Part model, mm, in its own coordinate system. A direction names the side the tool comes from. Round coordinates to 2 decimals unless told otherwise and drop trailing zeros. Write each loop counter-clockwise with the first axis right and the second up, starting at its lowest first coordinate (ties: lowest second). Pieces come first, ordered by that corner, then holes. Notation, with made-up numbers: M 29,32 L 80,32 A25 cw 80,57 Z; hole C -17.75,-20 d7. An arc over 180 degrees is marked long. One line per question, with ' | ' between items. Start each with the question number.
1) Tool access for faces 4 (the face through (-63.86, -11.924, 1.268)), 5 (the face through (-61.36, -7.4, -1.52)), 6 (the face through (-32.733, 21.384, 1.268)): list every direction of +Z, -Z, +X, -X, +Y, -Y with a clear straight run to the whole face (end or side of a thin tool).
2) Drop flat-ended pins along their axis: pin 1 Ø5 at (x, y) = (-45.06, 0.94) entering from +Z; pin 2 Ø3 at (x, y) = (-45.5, 13) entering from -Z; pin 3 Ø1.2 at (x, z) = (-39.5, 1.5) entering from +Y; pin 4 Ø4 at (x, y) = (-36.06, -17.06) entering from +Z. Give the stop position or say it passes through.
3) Saw through at C-C (y = 21). List the corners of the cut face in (x, z).
4) Mould opens along Y. For faces 1 (the face through (-45, 32, 0)), 2 (the face through (-61.36, 21.27, -1.52)), 3 (the face through (-45, -13.064, 1)) say: pulls with the +Y half, pulls with the -Y half, needs draft (parallel to the pull), parting line crosses it, or undercut.
5) Saw through at D-D (x = -48.5). List the corners of the cut face in (y, z), plus the area to 3 significant figures.
6) Saw through at A-A (x = -36). List the corners of the cut face in (y, z), plus the area to 3 significant figures.
7) Saw through at B-B (z = 0.65). List the corners of the cut face in (x, y).
8) Wall check: probe 1 along Y at (x, z) = (-44, -1.25); probe 2 along X at (y, z) = (19.5, -1.15); probe 3 along Y at (x, z) = (-32.5, 0.4). Give the ranges that are in metal, low to high. Write a range as [from, to].
```python
from build123d import *

# Parameters (mm, degrees)
SKETCH_2_W               = 40
SKETCH_2_H               = 40
EXTRUDE_1_DEPTH          = 2.5
SKETCH_5_W               = 40
SKETCH_5_H               = 60
SKETCH_5_R               = 1.5
EXTRUDE_2_DEPTH          = 3
SKETCH_4_R               = 1.5
SKETCH_4_R_2             = 1.10000034
CUT_EXTRUDE_1_DEPTH      = 6.5
FILLET_1_R               = 4
FILLET_5_R               = 2
SKETCH_6_R               = 3
CUT_EXTRUDE_2_DEPTH      = 3
MIRROR_2_COPY_1_SKETCH_R = 3
MIRROR_2_COPY_1_DEPTH    = 3
SKETCH_7_R               = 2
CUT_EXTRUDE_3_DEPTH      = 3


with BuildPart() as part:
    # 草图2 → 凸台-拉伸1 (new body)
    with BuildSketch(Plane.XY):
        with Locations((-45.062828034, 6.935543198)):
            Rectangle(SKETCH_2_W, SKETCH_2_H)
    extrude(amount=EXTRUDE_1_DEPTH)

    # 草图5 → 凸台-拉伸2 (add)
    with BuildSketch(Plane(origin=(0, 0, 0), x_dir=(-1, 0, 0), z_dir=(0, 0, -1))):
        with Locations((45.062828034, 6.935543198)):
            Rectangle(SKETCH_5_W, SKETCH_5_H)
        with Locations((36.062828034, 30.935543198)):
            Circle(SKETCH_5_R, mode=Mode.SUBTRACT)
        with Locations((54.062828034, 30.935543198)):
            Circle(SKETCH_5_R, mode=Mode.SUBTRACT)
        with Locations((54.062828034, -17.064456802)):
            Circle(SKETCH_5_R, mode=Mode.SUBTRACT)
        with Locations((36.062828034, -17.064456802)):
            Circle(SKETCH_5_R, mode=Mode.SUBTRACT)
    extrude(amount=EXTRUDE_2_DEPTH)

    # 草图4 → 切除-拉伸1 (cut, through all)
    with BuildSketch(Plane.XY.offset(2.5)):
        with Locations((-31.627799192, 20.370572041)):
            Circle(SKETCH_4_R)
        with Locations((-58.497856877, 20.370572041)):
            Circle(SKETCH_4_R)
        with Locations((-58.497856877, -6.499485644)):
            Circle(SKETCH_4_R)
        with Locations((-31.627799192, -6.499485644)):
            Circle(SKETCH_4_R)
        with Locations((-45.062828034, 12.935531198)):
            Circle(SKETCH_4_R_2)
        with Locations((-45.062828034, 0.935555198)):
            Circle(SKETCH_4_R_2)
    extrude(amount=-CUT_EXTRUDE_1_DEPTH, mode=Mode.SUBTRACT)

    # 圆角1
    fillet_1_edges = [part.edges().sort_by_distance(p)[0] for p in [
        (-25.062828034, -13.064456802, 1.25),
        (-65.062828034, -13.064456802, 1.25),
        (-65.062828034, 26.935543198, 1.25),
        (-25.062828034, 26.935543198, 1.25),
    ]]
    fillet(fillet_1_edges, radius=FILLET_1_R)

    # 圆角5
    fillet_5_edges = [part.edges().sort_by_distance(p)[0] for p in [
        (-25.062828034, 36.935543198, -1.5),
        (-25.062828034, -23.064456802, -1.5),
        (-65.062828034, -23.064456802, -1.5),
        (-65.062828034, 36.935543198, -1.5),
    ]]
    fillet(fillet_5_edges, radius=FILLET_5_R)

    # 草图6 → 切除-拉伸2 (cut)
    with BuildSketch(Plane(origin=(0, 0, -3), x_dir=(-1, 0, 0), z_dir=(0, 0, -1))):
        with Locations((58.497856877, 20.370572041)):
            Circle(SKETCH_6_R)
    cut_extrude_2 = extrude(amount=-CUT_EXTRUDE_2_DEPTH, mode=Mode.SUBTRACT)

    # 镜向1: 切除-拉伸2 across plane
    add(cut_extrude_2.mirror(Plane.ZX.offset(6.935543198)), mode=Mode.SUBTRACT)

    # 镜向2: 切除-拉伸2 across plane
    add(cut_extrude_2.mirror(Plane.ZY.offset(45.062828034)), mode=Mode.SUBTRACT)

    # 镜向2 copy 1 sketch → 镜向2 copy 1 (cut)
    with BuildSketch(Plane(origin=(-90.125656068, 13.871086397, -3), x_dir=(1, 0, 0), z_dir=(0, 0, -1))):
        with Locations((58.497856877, 20.370572041)):
            Circle(MIRROR_2_COPY_1_SKETCH_R)
    extrude(amount=-MIRROR_2_COPY_1_DEPTH, mode=Mode.SUBTRACT)

    # 草图7 → 切除-拉伸3 (cut)
    with BuildSketch(Plane(origin=(0, 0, -3), x_dir=(-1, 0, 0), z_dir=(0, 0, -1))):
        with Locations((45.062828034, 12.935531198)):
            Circle(SKETCH_7_R)
        with Locations((45.062828034, 0.935555198)):
            Circle(SKETCH_7_R)
    extrude(amount=-CUT_EXTRUDE_3_DEPTH, mode=Mode.SUBTRACT)


solid = part.part
```
Answer key:
1) face 4: +Z, -X, -Y | face 5: -Z | face 6: +Z, -Z
2) pin 1: stops at z = 2.5 | pin 2: stops at z = 0 | pin 3: stops at y = 26.94 | pin 4: stops at z = 0
3) outline: M -65.06,-3 L -61.43,-3 L -61.43,0 L -59.86,0 L -59.86,2.5 L -65.06,2.5 Z; M -57.14,0 L -55.56,0 L -55.56,-3 L -34.56,-3 L -34.56,0 L -32.99,0 L -32.99,2.5 L -57.14,2.5 Z; M -30.27,0 L -28.69,0 L -28.69,-3 L -25.06,-3 L -25.06,2.5 L -30.27,2.5 Z
4) face 1: needs draft | face 2: undercut | face 3: pulls with the -Y half
5) outline: M -23.06,-3 L 36.94,-3 L 36.94,0 L 26.94,0 L 26.94,2.5 L -13.06,2.5 L -13.06,0 L -23.06,0 Z | area: 280 mm2
6) outline: M -23.06,-3 L -18.56,-3 L -18.56,0 L -23.06,0 Z; M -15.57,-3 L 29.44,-3 L 29.44,0 L 26.94,0 L 26.94,2.5 L -13.06,2.5 L -13.06,0 L -15.57,0 Z; M 32.43,-3 L 36.94,-3 L 36.94,0 L 32.43,0 Z | area: 262 mm2
7) outline: M -65.06,-9.06 A4 ccw -61.06,-13.06 L -29.06,-13.06 A4 ccw -25.06,-9.06 L -25.06,22.94 A4 ccw -29.06,26.94 L -61.06,26.94 A4 ccw -65.06,22.94 Z; hole C -58.5,-6.5 d3; hole C -58.5,20.37 d3; hole C -45.06,0.94 d2.2; hole C -45.06,12.94 d2.2; hole C -31.63,-6.5 d3; hole C -31.63,20.37 d3
8) probe 1: y = [-23.06, -0.76], [2.63, 11.24], [14.63, 36.94] | probe 2: x = [-65.06, -61.37], [-55.63, -34.5], [-28.76, -25.06] | probe 3: y = [-13.06, -7.72], [-5.28, 19.15], [21.59, 26.94]
